```python
from build123d import *

# Parameters (mm, degrees)
BOSS_EXTRUDE1_DEPTH = 20
SKETCH6_W           = 5
SKETCH6_H           = 20
CUT_EXTRUDE1_DEPTH  = 293.280687012
SKETCH7_R           = 1.5
BOSS_EXTRUDE2_DEPTH = 15
BOSS_EXTRUDE3_START = 15
SKETCH8_R           = 1.5
BOSS_EXTRUDE3_DEPTH = 15


with BuildPart() as part:
    # Sketch5 → Boss-Extrude1 (new body)
    with BuildSketch(Plane.XY):
        Polygon((0, 0), (-42.5, 0), (-131, -108), (-131, -128), (-128, -128), (-128, -109.072168564), (-41.07975076, -3), (0, -3), align=None)
        Polygon((42.5, 0), (0, 0), (0, -3), (41.07975076, -3), (128, -109.072168564), (128, -128), (131, -128), (131, -108), align=None)
    extrude(amount=BOSS_EXTRUDE1_DEPTH)

    # Sketch6 → Cut-Extrude1 (cut, through all)
    with BuildSketch(Plane(origin=(131, 0, 0), x_dir=(0, 0, -1), z_dir=(1, 0, 0))):
        with Locations((-17.5, -118)):
            Rectangle(SKETCH6_W, SKETCH6_H)
        Polygon((-20, -108), (-15, -108), (-20, 0), align=None)
        Polygon((0, 0), (-5, -108), (0, -108), align=None)
        with Locations((-2.5, -118)):
            Rectangle(SKETCH6_W, SKETCH6_H)
    extrude(amount=-CUT_EXTRUDE1_DEPTH, mode=Mode.SUBTRACT)

    # Sketch7 → Boss-Extrude2 (add)
    with BuildSketch(Plane(origin=(131, 0, 0), x_dir=(0, 0, -1), z_dir=(1, 0, 0))):
        with Locations((-10, -123)):
            Circle(SKETCH7_R)
    extrude(amount=BOSS_EXTRUDE2_DEPTH)

    # Sketch8 → Boss-Extrude3 (add)
    with BuildSketch(Plane.ZY.offset(131).offset(BOSS_EXTRUDE3_START)):
        with Locations(Location((10, -123, 0), (0, 0, 180))):
            Circle(SKETCH8_R)
    extrude(amount=-BOSS_EXTRUDE3_DEPTH)


solid = part.part
```
Geometry check sheet. Reference: the model listing, model coordinates, mm. A direction names the side the tool comes from. Give positions to 0.01 mm unless a question says otherwise; leave off trailing zeros. Loops run counter-clockwise (first coordinate to the right, second up) from the corner with the lowest first, then second, coordinate; pieces in that order, holes last. Notation, with made-up numbers: M -29.75,0.25 L 17.25,0.25 A20 cw 17.25,19.25 Z; hole C 7,41 d11. An arc over 180 degrees is marked long. Write item = value, one per line.
(1) Release check for a two-part mould opening along X. For faces 3 (the face through (1, 0, 10)), 4 (the face through (74.274, -43.508, 9.862)), 5 (the face through (-131, -118, 10)) record: released by +X, released by -X, zero draft, split by the parting line, or undercut.
Answer below:
face_3 = zero draft
face_4 = undercut
face_5 = released by -X
(2) Sectioned sample at C-C, the plane x = -8.5. Record the cut outline in (y, z).
Answer below:
outline = M -3,0.14 L 0,0 L 0,20 L -3,19.86 Z
(3) Sectioned sample at D-D, the plane x = 117.5. Record the cut outline in (y, z).
Answer below:
outline = M -96.26,4.46 L -91.53,4.24 L -91.53,15.76 L -96.26,15.54 Z
(4) Sectioned sample at A-A, the plane y = -91. Record the cut outline in (x, z), plus the area to 3 significant figures.
Answer below:
outline = M -117.07,4.21 L -113.19,4.21 L -113.19,15.79 L -117.07,15.79 Z; M 113.19,4.21 L 117.07,4.21 L 117.07,15.79 L 113.19,15.79 Z
area = 89.8 mm2
(5) Material ranges on line 1 (X direction, y = -115.5, z = 10.25); line 2 (X direction, y = -28.5, z = 8); line 3 (Y direction, x = 98, z = 9), recorded low to high. Write a range as [from, to].
Answer below:
line_1 = [-131, -128], [128, 131]
line_2 = [-65.85, -61.98], [61.98, 65.85]
line_3 = [-72.46, -67.73]
(6) Tool access check on faces 1 (the face through (77.54, -42.76, 9.86)), 2 (the face through (-1, -3, 10)). Record the directions out of +Z, -Z, +X, -X, +Y, -Y that give a thin tool (end or side, any length) a straight path to the whole face; none if there is none.
Answer below:
face_1 = +Z, -Z, +X, +Y
face_2 = +Z, -Z, -Y
(7) Gauge pin test, flat ends, axial feed: pin 1 Ø1.9 at (x, y) = (130, -117.5) entering from +Z; pin 2 Ø1.9 at (x, y) = (-128, -120.5) entering from -Z; pin 3 Ø3 at (x, z) = (52, 5.5) entering from -Y; pin 4 Ø2 at (y, z) = (-94, 2) entering from -X. Record the tip position at first contact, or that the pin passes through.
Answer below:
pin_1 = 15
pin_2 = 5
pin_3 = -18.16
pin_4 = through
(8) Sectioned sample at B-B, the plane y = -74. Record the cut outline in (x, z), plus the area to 3 significant figures.
Answer below:
outline = M -103.14,3.43 L -99.26,3.43 L -99.26,16.57 L -103.14,16.57 Z; M 99.26,3.43 L 103.14,3.43 L 103.14,16.57 L 99.26,16.57 Z
area = 102 mm2
